The model under review builds one solid part; all positions refer to its coordinate system, in mm. Face numbers are marked on the shaded views. Round coordinates to 2 decimals unless told otherwise and drop trailing zeros. Order: outer loops, then holes, each group sorted by start corner. A loop starts at its lowest first (then second) coordinate and runs counter-clockwise, first axis right, second up. Notation, with made-up numbers: (-39.5, -35.75) -> (9.5, -35.75) arc R25 ccw to (9.5, -4.75) -> close; hole circle Ø10 at (70, 33). An arc over 180 degrees is marked (long way). Use a Markdown table: item, result. Add a question column.
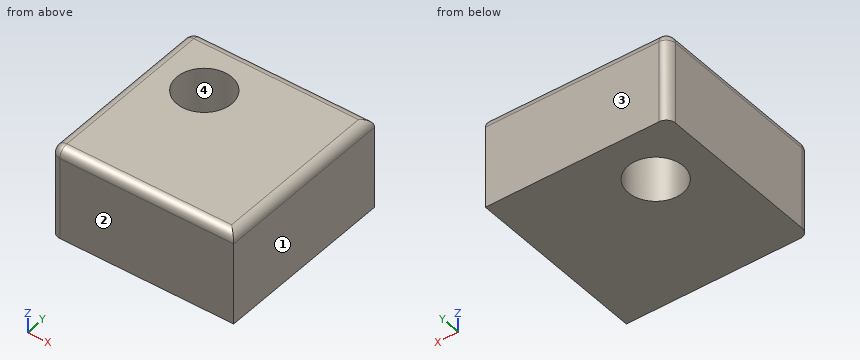
```python
from build123d import *

# Parameters (mm, degrees)
F0_W     = 100
F0_H     = 100
F1_DEPTH = 50
F2_R     = 15
F3_DEPTH = 50.001
F4_R     = 5
F5_R     = 5


with BuildPart() as f1:
    # F0 (on Top) → F1 (new body)
    with BuildSketch(Plane.XY):
        Rectangle(F0_W, F0_H)
    extrude(amount=F1_DEPTH)

    # F2 (on face) → F3 (cut, through all)
    with BuildSketch(Plane.XY.offset(50)):
        with Locations((-20, 20)):
            Circle(F2_R)
    extrude(amount=-F3_DEPTH, mode=Mode.SUBTRACT)

    # F4
    f4_edges = [f1.edges().sort_by_distance(p)[0] for p in [
        (-50, 0, 50),
    ]]
    fillet(f4_edges, radius=F4_R)

    # F5
    f5_edges = [f1.edges().sort_by_distance(p)[0] for p in [
        (2.5, -50, 50),
        (50, 0, 50),
        (2.5, 50, 50),
    ]]
    fillet(f5_edges, radius=F5_R)


solid = f1.part
```
Q1. Add section B-B, the plane y = 20. Give the boundary of the cut face in (x, z).
Q2. To check wall thickness, follow line 1 along Y through (x, z) = (-20, 22); line 2 along Z through (x, y) = (45.5, -19); line 3 along X through (y, z) = (10.5, 10). State the ranges of each line that lie inside material, in increasing order.
Q3. Add section C-C, the plane z = 6.5. Give the boundary of the cut face in (x, y).
Q4. Add section A-A, the plane x = -20. Give the boundary of the cut face in (y, z), then the cut area to 3 significant figures.
Q5. Draft analysis for pull direction Y (two halves, no side actions). For the marked faces 1, 2, 3 and 4, state which applies: released by +Y, released by -Y, zero draft, split by the parting line, or undercut.
Return value:
| question | item | result |
|---|---|---|
| 1 | outline | (-50, 0) -> (-35, 0) -> (-35, 50) -> (-45, 50) arc R5 ccw to (-50, 45) -> close; (-5, 0) -> (50, 0) -> (50, 45) arc R5 ccw to (45, 50) -> (-5, 50) -> close |
| 2 | line 1 | -50 to 5, 35 to 50 |
| 2 | line 2 | 0 to 49.97 |
| 2 | line 3 | -50 to -31.61, -8.39 to 50 |
| 3 | outline | (-50, -45) arc R5 ccw to (-45, -50) -> (50, -50) -> (50, 50) -> (-45, 50) arc R5 ccw to (-50, 45) -> close; hole circle Ø30 at (-20, 20) |
| 4 | outline | (-50, 0) -> (5, 0) -> (5, 50) -> (-45, 50) arc R5 ccw to (-50, 45) -> close; (35, 0) -> (50, 0) -> (50, 45) arc R5 ccw to (45, 50) -> (35, 50) -> close |
| 4 | area | 3,490 mm² |
| 5 | face 1 | zero draft |
| 5 | face 2 | released by -Y |
| 5 | face 3 | released by +Y |
| 5 | face 4 | undercut |
